Design review of the part built by this model. Coordinates are the model's own, in mm. A direction names the side the tool comes from. Give positions to 0.01 mm unless a question says otherwise; leave off trailing zeros. Order: outer loops, then holes, each group sorted by start corner. A loop starts at its lowest first (then second) coordinate and runs counter-clockwise, first axis right, second up. Notation, with made-up numbers: (24.25, 20) -> (79.25, 20) arc R13 cw to (79.25, 31) -> close; hole circle Ø9 at (14, 26.5). An arc over 180 degrees is marked (long way). Use a Markdown table: item, result. Add a question column.
```python
from build123d import *

# Parameters (mm, degrees)
SKETCH_1_R          = 12.25
EXTRUDE_1_DEPTH     = 2
SKETCH_2_R          = 4
EXTRUDE_2_DEPTH     = 3
SKETCH_3_R          = 1.25
CUT_EXTRUDE_1_DEPTH = 3
SKETCH_4_R          = 3
CUT_EXTRUDE_2_DEPTH = 3


with BuildPart() as part:
    # 草图1 → 凸台-拉伸1 (new body)
    with BuildSketch(Plane(origin=(0, 0, 0), x_dir=(1, 0, 0), z_dir=(0, 1, 0))):
        with Locations(Location((0, 0, 0), (0, 0, 270))):
            Circle(SKETCH_1_R)
    extrude(amount=EXTRUDE_1_DEPTH)

    # 草图2 → 凸台-拉伸2 (add)
    with BuildSketch(Plane(origin=(0, 2, 0), x_dir=(1, 0, 0), z_dir=(0, 1, 0))):
        with Locations(Location((0, 0, 0), (0, 0, 270))):
            Circle(SKETCH_2_R)
    extrude(amount=EXTRUDE_2_DEPTH)

    # 草图3 → 切除-拉伸1 (cut)
    with BuildSketch(Plane(origin=(0, 2, 0), x_dir=(1, 0, 0), z_dir=(0, 1, 0))):
        with Locations(Location((-8, 0, 0), (0, 0, 270))):
            Circle(SKETCH_3_R)
        with Locations(Location((0, 8, 0), (0, 0, 270))):
            Circle(SKETCH_3_R)
        with Locations(Location((8, 0, 0), (0, 0, 270))):
            Circle(SKETCH_3_R)
        with Locations(Location((0, -8, 0), (0, 0, 270))):
            Circle(SKETCH_3_R)
    extrude(amount=-CUT_EXTRUDE_1_DEPTH, mode=Mode.SUBTRACT)

    # 草图4 → 切除-拉伸2 (cut)
    with BuildSketch(Plane(origin=(0, 5, 0), x_dir=(1, 0, 0), z_dir=(0, 1, 0))):
        with Locations(Location((0, 0, 0), (0, 0, 270))):
            Circle(SKETCH_4_R)
    extrude(amount=-CUT_EXTRUDE_2_DEPTH, mode=Mode.SUBTRACT)


solid = part.part
```
1) Machinability: for faces 1 (the flat face through (0, 0, 0)), 2 (the cylindrical face through (0.9, 3.52, 2.86)), which of the approach directions +Z, -Z, +X, -X, +Y, -Y give a long, thin tool a straight path to every point of the face, cutting with its end or side? Answer none if there is none.
2) Insertion check: pin 1 (2 mm diameter, centred on x = 9, z = -5, fed in from -Y); pin 2 (2 mm diameter, centred on y = 0.5, z = -6.5, fed in from -X); pin 3 (1 mm diameter, centred on y = 2, z = 5.5, fed in from -X); pin 4 (4 mm diameter, centred on x = 8, z = 0, fed in from +Y). Each pin has a flat end and moves straight along its axis. Give the tip position at first contact, or say it passes through.
3) The part is to be moulded in two halves that separate along Z. For faces 3 (the flat face through (3, 2, -3)), 4 (the cylindrical face through (-9.22, 1.01, -0.27)), 5 (the cylindrical face through (3.68, 0.986, 11.684)), say which applies: +Z half, -Z half, draft (parallel to the pull), parting line (faces both ways), or undercut.
4) Add section C-C (y = 1.7). Give the boundary of the cut face in (x, z).
5) Add section B-B (z = -8). Give the boundary of the cut face in (x, y), then the cut area to 3 significant figures.
6) For L1, parallel to X at y = 0.6, z = 0; L2, parallel to X at y = 3.6, z = 0; L3, parallel to Y at x = -4.75, z = 6.5, list the stretches that pass through material, from the lowest coordinate up. Write a range as [from, to].
7) Add section D-D (x = 8). Give the boundary of the cut face in (y, z).
8) Add section A-A (x = 0). Give the boundary of the cut face in (y, z), then the cut area to 3 significant figures.
Worked answers:
| question | item | result |
|---|---|---|
| 1 | face 1 | +Z, -Z, +X, -X, -Y |
| 1 | face 2 | +Y |
| 2 | pin 1 | y = 0 |
| 2 | pin 2 | x = -10.95 |
| 2 | pin 3 | x = -11.18 |
| 2 | pin 4 | y = 2 |
| 3 | face 3 | draft |
| 3 | face 4 | undercut |
| 3 | face 5 | parting line |
| 4 | outline | circle Ø24.5 at (0, 0); hole circle Ø2.5 at (-8, 0); hole circle Ø2.5 at (0, -8); hole circle Ø2.5 at (0, 8); hole circle Ø2.5 at (8, 0) |
| 5 | outline | (-9.28, 0) -> (-1.25, 0) -> (-1.25, 2) -> (-9.28, 2) -> close; (1.25, 0) -> (9.28, 0) -> (9.28, 2) -> (1.25, 2) -> close |
| 5 | area | 32.1 mm^2 |
| 6 | L1 | [-12.25, -9.25], [-6.75, 6.75], [9.25, 12.25] |
| 6 | L2 | [-4, -3], [3, 4] |
| 6 | L3 | [0, 2] |
| 7 | outline | (0, -9.28) -> (2, -9.28) -> (2, -1.25) -> (0, -1.25) -> close; (0, 1.25) -> (2, 1.25) -> (2, 9.28) -> (0, 9.28) -> close |
| 8 | outline | (0, -12.25) -> (2, -12.25) -> (2, -9.25) -> (0, -9.25) -> close; (0, -6.75) -> (2, -6.75) -> (2, -4) -> (5, -4) -> (5, -3) -> (2, -3) -> (2, 3) -> (5, 3) -> (5, 4) -> (2, 4) -> (2, 6.75) -> (0, 6.75) -> close; (0, 9.25) -> (2, 9.25) -> (2, 12.25) -> (0, 12.25) -> close |
| 8 | area | 45.0 mm^2 |
